```python
from build123d import *

# Parameters (mm, degrees)
F0_R     = 12.7
F1_DEPTH = 5.842
F3_DEPTH = 5.842
F4_DEPTH = 25.4


with BuildPart() as f1:
    # F0 (on Top) → F1 (new body)
    with BuildSketch(Plane.XY):
        Circle(F0_R)
    extrude(amount=F1_DEPTH)

    # F2 (on face) → F3 (join)
    with BuildSketch(Plane.XY.offset(5.842)):
        with BuildLine():
            ThreePointArc((4.678035, 11.807031), (4.741337, 12.251523), (4.7625, 12.7))
            ThreePointArc((4.7625, 12.7), (-0.448477, 17.441337), (-4.678035, 11.807031))
            ThreePointArc((-4.678035, 11.807031), (-3.463658, 12.218554), (-2.213976, 12.505531))
            ThreePointArc((-2.213976, 12.505531), (-0.097328, 14.920368), (2.2225, 12.7))
            ThreePointArc((2.2225, 12.7), (2.220368, 12.602672), (2.213976, 12.505531))
            ThreePointArc((2.213976, 12.505531), (3.463658, 12.218554), (4.678035, 11.807031))
        make_face()
    extrude(amount=-F3_DEPTH)

    # F2 (on face) → F4 (cut)
    with BuildSketch(Plane.XY.offset(5.842)):
        with BuildLine():
            ThreePointArc((2.213976, 12.505531), (0, 12.7), (-2.213976, 12.505531))
            ThreePointArc((-2.213976, 12.505531), (0, 10.4775), (2.213976, 12.505531))
        make_face()
    extrude(amount=-F4_DEPTH, mode=Mode.SUBTRACT)


solid = f1.part
```
Build history of the part. All positions in model axes, mm. Round coordinates to 2 decimals unless told otherwise and drop trailing zeros. Loops run counter-clockwise (first coordinate to the right, second up) from the corner with the lowest first, then second, coordinate; pieces in that order, holes last.
Item 1: Pin check, flat tips, straight feed: P1, Ø2, axis at y = 6, z = 5, coming from the +X side; P2, Ø8, axis at x = 4, y = 9, coming from the -Z side; P3, Ø1, axis at y = 6, z = 1.5, coming from the -X side. Stop position of each tip, or through.
Item 2: Drill centre lines: line 1 along X through (y, z) = (12.5, 4.2); line 2 along X through (y, z) = (11, 5.2); line 3 along Y through (x, z) = (-1, 1.45). Where is each one in solid material? Low to high.
Item 3: Saw through at A-A (x = 0). List the corners of the cut face in (y, z).
Item 4: Two-plate mould, pull along Y, no slides. Class faces 1 (the face through (0, 3, 0)), 2 (the face through (4.74, 12.25, 2.96)): released by +Y, released by -Y, zero draft, split by the parting line, or undercut.
Item 5: Saw through at C-C (y = -10.5). List the corners of the cut face in (x, z), then the cut area to 3 significant figures.
Item 6: Saw through at D-D (x = -7.5). List the corners of the cut face in (y, z), then the cut area to 3 significant figures.
Worked answers:
1. P1: stops at x = 11.67
1. P2: stops at z = 0
1. P3: stops at x = -11.45
2. line 1: x = -4.76 to -2.21, 2.21 to 4.76
2. line 2: x = -6.35 to -1.43, 1.43 to 6.35
2. line 3: y = -12.66 to 10.72, 14.68 to 17.36
3. outline: (-12.7, 0) - (10.48, 0) - (10.48, 5.84) - (-12.7, 5.84) - close; (14.92, 0) - (17.46, 0) - (17.46, 5.84) - (14.92, 5.84) - close
4. face 1: zero draft
4. face 2: undercut
5. outline: (-7.14, 0) - (7.14, 0) - (7.14, 5.84) - (-7.14, 5.84) - close
5. area: 83.5 mm2
6. outline: (-10.25, 0) - (10.25, 0) - (10.25, 5.84) - (-10.25, 5.84) - close
6. area: 120 mm2
